Check sheet for the modelled part. Datum: model origin and axes. Units: mm. A direction names the side the tool comes from. Coordinates: 2 decimals unless noted, no trailing zeros. Loops run counter-clockwise (first coordinate to the right, second up) from the corner with the lowest first, then second, coordinate; pieces in that order, holes last.
```python
from build123d import *

# Parameters (mm, degrees)
SKETCH1_W           = 50.8
SKETCH1_H           = 25.4
SKETCH1_W_2         = 47.625
SKETCH1_H_2         = 22.225
BOSS_EXTRUDE1_DEPTH = 177.8
CUT_EXTRUDE1_REACH  = 183.392
SKETCH2_W           = 25.4
SKETCH2_H           = 50.8


with BuildPart() as part:
    # Sketch1 → Boss-Extrude1 (new body)
    with BuildSketch(Plane.XY):
        Rectangle(SKETCH1_W, SKETCH1_H)
        Rectangle(SKETCH1_W_2, SKETCH1_H_2, mode=Mode.SUBTRACT)
    extrude(amount=BOSS_EXTRUDE1_DEPTH)

    # Cut-Extrude1: up to this face of the body (flat: up to its plane)
    cut_extrude1_end = Plane(part.part.faces().sort_by_distance((0, -12.7, 88.9))[0])
    # Sketch2 → Cut-Extrude1 (cut, up to the picked face)
    with BuildSketch(Plane(origin=(0, 12.7, 0), x_dir=(1, 0, 0), z_dir=(0, 1, 0)), mode=Mode.PRIVATE) as cut_extrude1_sk1:
        with BuildLine():
            ThreePointArc((-25.4, -25.4), (-17.960512214, -7.439487729), (8.1e-08, 0))
            Line((8.1e-08, 0), (-25.4, 0))
            Line((-25.4, 0), (-25.4, -25.4))
        make_face()
    cut_extrude1_tool1 = split(extrude(cut_extrude1_sk1.sketch, amount=-CUT_EXTRUDE1_REACH, mode=Mode.PRIVATE), bisect_by=cut_extrude1_end, keep=Keep.BOTH, mode=Mode.PRIVATE)
    # Sketch2 → Cut-Extrude1 (cut, up to the picked face)
    with BuildSketch(Plane(origin=(0, 12.7, 0), x_dir=(1, 0, 0), z_dir=(0, 1, 0)), mode=Mode.PRIVATE) as cut_extrude1_sk2:
        with BuildLine():
            ThreePointArc((-19.05, -25.4), (0, -44.45), (19.05, -25.4))
            Line((19.05, -25.4), (-19.05, -25.4))
        make_face()
    cut_extrude1_tool2 = split(extrude(cut_extrude1_sk2.sketch, amount=-CUT_EXTRUDE1_REACH, mode=Mode.PRIVATE), bisect_by=cut_extrude1_end, keep=Keep.BOTH, mode=Mode.PRIVATE)
    # Sketch2 → Cut-Extrude1 (cut, up to the picked face)
    with BuildSketch(Plane(origin=(0, 12.7, 0), x_dir=(1, 0, 0), z_dir=(0, 1, 0)), mode=Mode.PRIVATE) as cut_extrude1_sk3:
        with BuildLine():
            Line((-19.05, -25.4), (19.05, -25.4))
            ThreePointArc((19.05, -25.4), (0, -6.35), (-19.05, -25.4))
        make_face()
    cut_extrude1_tool3 = split(extrude(cut_extrude1_sk3.sketch, amount=-CUT_EXTRUDE1_REACH, mode=Mode.PRIVATE), bisect_by=cut_extrude1_end, keep=Keep.BOTH, mode=Mode.PRIVATE)
    # Sketch2 → Cut-Extrude1 (cut, up to the picked face)
    with BuildSketch(Plane(origin=(0, 12.7, 0), x_dir=(1, 0, 0), z_dir=(0, 1, 0)), mode=Mode.PRIVATE) as cut_extrude1_sk4:
        with BuildLine():
            ThreePointArc((8.1e-08, 0), (17.960512271, -7.439487786), (25.4, -25.4))
            Line((25.4, -25.4), (25.4, 0))
            Line((25.4, 0), (8.1e-08, 0))
        make_face()
    cut_extrude1_tool4 = split(extrude(cut_extrude1_sk4.sketch, amount=-CUT_EXTRUDE1_REACH, mode=Mode.PRIVATE), bisect_by=cut_extrude1_end, keep=Keep.BOTH, mode=Mode.PRIVATE)
    # Sketch2 → Cut-Extrude1 (cut, up to the picked face)
    with BuildSketch(Plane(origin=(0, 12.7, 0), x_dir=(1, 0, 0), z_dir=(0, 1, 0)), mode=Mode.PRIVATE) as cut_extrude1_sk5:
        with BuildLine():
            ThreePointArc((-19.05, -25.4), (0, -44.45), (19.05, -25.4))
            Line((19.05, -25.4), (-19.05, -25.4))
        make_face()
    cut_extrude1_tool5 = split(extrude(cut_extrude1_sk5.sketch, amount=-CUT_EXTRUDE1_REACH, mode=Mode.PRIVATE), bisect_by=cut_extrude1_end, keep=Keep.BOTH, mode=Mode.PRIVATE)
    # Sketch2 → Cut-Extrude1 (cut, up to the picked face)
    with BuildSketch(Plane(origin=(0, 12.7, 0), x_dir=(1, 0, 0), z_dir=(0, 1, 0)), mode=Mode.PRIVATE) as cut_extrude1_sk6:
        with BuildLine():
            Line((-19.05, -25.4), (19.05, -25.4))
            ThreePointArc((19.05, -25.4), (0, -6.35), (-19.05, -25.4))
        make_face()
    cut_extrude1_tool6 = split(extrude(cut_extrude1_sk6.sketch, amount=-CUT_EXTRUDE1_REACH, mode=Mode.PRIVATE), bisect_by=cut_extrude1_end, keep=Keep.BOTH, mode=Mode.PRIVATE)
    # Sketch2 → Cut-Extrude1 (cut, up to the picked face)
    with BuildSketch(Plane(origin=(0, 12.7, 0), x_dir=(1, 0, 0), z_dir=(0, 1, 0)), mode=Mode.PRIVATE) as cut_extrude1_sk7:
        with Locations((0, -133.35)):
            Rectangle(SKETCH2_W, SKETCH2_H)
    cut_extrude1_tool7 = split(extrude(cut_extrude1_sk7.sketch, amount=-CUT_EXTRUDE1_REACH, mode=Mode.PRIVATE), bisect_by=cut_extrude1_end, keep=Keep.BOTH, mode=Mode.PRIVATE)
    # Sketch2 → Cut-Extrude1 (cut, up to the picked face)
    with BuildSketch(Plane(origin=(0, 12.7, 0), x_dir=(1, 0, 0), z_dir=(0, 1, 0)), mode=Mode.PRIVATE) as cut_extrude1_sk8:
        with Locations((0, -76.2)):
            Rectangle(SKETCH2_W, SKETCH2_H)
    cut_extrude1_tool8 = split(extrude(cut_extrude1_sk8.sketch, amount=-CUT_EXTRUDE1_REACH, mode=Mode.PRIVATE), bisect_by=cut_extrude1_end, keep=Keep.BOTH, mode=Mode.PRIVATE)
    add(cut_extrude1_tool1.solids().sort_by(Axis((-19.726454, 12.7, 5.673546), (0, -1, 0)))[0], mode=Mode.SUBTRACT)
    add(cut_extrude1_tool2.solids().sort_by(Axis((0, 12.7, 33.485071), (0, -1, 0)))[0], mode=Mode.SUBTRACT)
    add(cut_extrude1_tool3.solids().sort_by(Axis((0, 12.7, 17.314929), (0, -1, 0)))[0], mode=Mode.SUBTRACT)
    add(cut_extrude1_tool4.solids().sort_by(Axis((19.726454, 12.7, 5.673546), (0, -1, 0)))[0], mode=Mode.SUBTRACT)
    add(cut_extrude1_tool5.solids().sort_by(Axis((0, 12.7, 33.485071), (0, -1, 0)))[0], mode=Mode.SUBTRACT)
    add(cut_extrude1_tool6.solids().sort_by(Axis((0, 12.7, 17.314929), (0, -1, 0)))[0], mode=Mode.SUBTRACT)
    add(cut_extrude1_tool7.solids().sort_by(Axis((0, 12.7, 133.35), (0, -1, 0)))[0], mode=Mode.SUBTRACT)
    add(cut_extrude1_tool8.solids().sort_by(Axis((0, 12.7, 76.2), (0, -1, 0)))[0], mode=Mode.SUBTRACT)


solid = part.part
```
1) Mould release check, pull along X, two halves, no side actions. Record for faces 1 (the flat face through (25.4, 0, 101)), 2 (the cylindrical face through (-2.48, -11.895, 6.512)), 3 (the flat face through (0, -12, 177.8)): +X half, -X half, draft (parallel to the pull), parting line (faces both ways), or undercut.
Answer sheet:
face 1: +X half
face 2: undercut
face 3: draft
2) Section check A-A on y = 4. Enter the section's corners in (x, z).
Answer sheet:
outline: (-25.4, 25.4) arc R25.4 ccw to (-23.81, 16.56) - (-23.81, 177.8) - (-25.4, 177.8) - close; (23.81, 16.56) arc R25.4 ccw to (25.4, 25.4) - (25.4, 177.8) - (23.81, 177.8) - close
3) Section check D-D on z = 12.5. Enter the section's corners in (x, y).
Answer sheet:
outline: (-21.88, -12.7) - (-14.02, -12.7) - (-14.02, -11.11) - (-21.88, -11.11) - close; (-21.88, 11.11) - (-14.02, 11.11) - (-14.02, 12.7) - (-21.88, 12.7) - close; (14.02, -12.7) - (21.88, -12.7) - (21.88, -11.11) - (14.02, -11.11) - close; (14.02, 11.11) - (21.88, 11.11) - (21.88, 12.7) - (14.02, 12.7) - close
4) Scan lines: line 1 (X direction, y = -11.65, z = 25.4); line 2 (X direction, y = 0.25, z = 100.5); line 3 (Y direction, x = 23, z = 35). Record each from-to range of solid material in increasing order.
Answer sheet:
line 1: x = -25.4 to -19.05, 19.05 to 25.4
line 2: x = -25.4 to -23.81, 23.81 to 25.4
line 3: y = -12.7 to -11.11, 11.11 to 12.7
5) Section check C-C on x = -22. Enter the section's corners in (y, z).
Answer sheet:
outline: (-12.7, 12.71) - (-11.11, 12.71) - (-11.11, 177.8) - (-12.7, 177.8) - close; (11.11, 12.71) - (12.7, 12.71) - (12.7, 177.8) - (11.11, 177.8) - close
6) Depth check by flat-ended pin: pin 1 (1.3 mm diameter, centred on x = -6, y = -12, fed in from -Z); pin 2 (8 mm diameter, centred on x = 6.5, y = 7.5, fed in from -Z); pin 3 (1 mm diameter, centred on y = -9, z = 18.5, fed in from -X); pin 4 (12 mm diameter, centred on x = -6.5, y = 4.5, fed in from -Z). Enter the tip coordinate at first touch or a pass-through.
Answer sheet:
pin 1: stops at z = 0.57
pin 2: stops at z = 0.45
pin 3: stops at x = -24.58
pin 4: passes through
7) Section check B-B on z = 140. Enter the section's corners in (x, y).
Answer sheet:
outline: (-25.4, -12.7) - (-12.7, -12.7) - (-12.7, -11.11) - (-23.81, -11.11) - (-23.81, 11.11) - (-12.7, 11.11) - (-12.7, 12.7) - (-25.4, 12.7) - close; (12.7, -12.7) - (25.4, -12.7) - (25.4, 12.7) - (12.7, 12.7) - (12.7, 11.11) - (23.81, 11.11) - (23.81, -11.11) - (12.7, -11.11) - close
8) Set-up check for faces 4 (the flat face through (0, 11.112, 107)), 5 (the cylindrical face through (-2.48, 11.917, 6.512)): record each of +Z, -Z, +X, -X, +Y, -Y from which the full face is reachable in a straight line by a thin tool's end or side.
Answer sheet:
face 4: +Z, -Z
face 5: +Y, -Y
